```python
from build123d import *

# Parameters (mm, degrees)
SKETCH1_W           = 25
SKETCH1_H           = 30
SKETCH1_R           = 1.5
SKETCH1_R_2         = 3.5
SKETCH1_W_2         = 30
SKETCH1_H_2         = 5
BOSS_EXTRUDE4_DEPTH = 3


with BuildPart() as part:
    # Sketch1 → Boss-Extrude4 (new body)
    # profile 1 of 2: a face of its own
    with BuildSketch(Plane(origin=(0, 0, 0), x_dir=(1, 0, 0), z_dir=(0, 1, 0))):
        with Locations((-26.523048167, -1.727371577)):
            Rectangle(SKETCH1_W, SKETCH1_H)
        with Locations(Location((-18.023048167, -1.727371577, 0), (0, 0, 270))):
            Circle(SKETCH1_R, mode=Mode.SUBTRACT)
        with Locations(Location((-26.523048167, -1.727371577, 0), (0, 0, 270))):
            Circle(SKETCH1_R_2, mode=Mode.SUBTRACT)
        with Locations(Location((-35.023048167, -1.727371577, 0), (0, 0, 270))):
            Circle(SKETCH1_R, mode=Mode.SUBTRACT)
    # profile 2 of 2: a face of its own
    with BuildSketch(Plane(origin=(0, 0, 0), x_dir=(1, 0, 0), z_dir=(0, 1, 0))):
        with Locations((-26.523048167, -19.227371577)):
            Rectangle(SKETCH1_W_2, SKETCH1_H_2)
    extrude(amount=BOSS_EXTRUDE4_DEPTH)


solid = part.part
```
Could you check a few things on this model? Use its own coordinates, in mm. A direction names the side the tool comes from. Coordinates: 2 decimals unless noted, no trailing zeros. Write each loop counter-clockwise with the first axis right and the second up, starting at its lowest first coordinate (ties: lowest second). Pieces come first, ordered by that corner, then holes. Notation, with made-up numbers: (-22.75, 73.5) -> (29.25, 73.5) arc R35 cw to (29.25, 111.5) -> close; hole circle Ø2 at (80.5, 38). An arc over 180 degrees is marked (long way). Return JSON: item names as keys, results as strings.
(1) We'd pull the mould along X, two halves only. Please class faces 4 (the flat face through (-27, 1, -13.273)), 5 (the cylindrical face through (-19.487, 1.479, 1.402)), 6 (the cylindrical face through (-33.536, 1.479, 1.532)), 7 (the flat face through (-11.523, 1, 19)): +X half, -X half, draft (parallel to the pull), parting line (faces both ways), or undercut.
Numbers:
{"face 4": "draft", "face 5": "undercut", "face 6": "undercut", "face 7": "+X half"}
(2) Imagine slicing it at D-D, the plane z = -9. Please give me the cut outline in (x, y), then the cut area to 3 significant figures.
Numbers:
{"outline": "(-39.02, 0) -> (-14.02, 0) -> (-14.02, 3) -> (-39.02, 3) -> close", "area": "75.0 mm2"}
(3) I'm going to push flat-ended pins straight in: pin 1 (1.5 mm diameter, centred on y = 1, z = 7.5, fed in from +X); pin 2 (0.8 mm diameter, centred on x = -12.5, y = 1.5, fed in from -Z); pin 3 (4 mm diameter, centred on x = -26.52, z = 1.73, fed in from +Y). Where does each tip first touch, or does it pass through?
Numbers:
{"pin 1": "stops at x = -14.02", "pin 2": "stops at z = 16.73", "pin 3": "passes through"}
(4) Which directions (+Z, -Z, +X, -X, +Y, -Y) give clear straight access to the entire face, cutting with the end or side of a thin tool? Please do faces 1 (the flat face through (-40, 1, 16.727)), 2 (the flat face through (-13, 1, 16.727)), 3 (the cylindrical face through (-23.053, 1.479, 1.272)).
Numbers:
{"face 1": "-Z, -X, +Y, -Y", "face 2": "-Z, +X, +Y, -Y", "face 3": "+Y, -Y"}
(5) Imagine slicing it at C-C, the plane x = -24.5. Please give me the cut outline in (y, z), then the cut area to 3 significant figures.
Numbers:
{"outline": "(0, -13.27) -> (3, -13.27) -> (3, -1.13) -> (0, -1.13) -> close; (0, 4.58) -> (3, 4.58) -> (3, 21.73) -> (0, 21.73) -> close", "area": "87.9 mm2"}
(6) Imagine slicing it at A-A, the plane z = 4.5. Please give me the cut outline in (x, y), then the cut area to 3 significant figures.
Numbers:
{"outline": "(-39.02, 0) -> (-28.66, 0) -> (-28.66, 3) -> (-39.02, 3) -> close; (-24.39, 0) -> (-14.02, 0) -> (-14.02, 3) -> (-24.39, 3) -> close", "area": "62.2 mm2"}
(7) I need wall thicknesses on L1, parallel to Z at x = -35, y = 2.2; L2, parallel to X at y = 2.6, z = 7; L3, parallel to Z at x = -13.5, y = 1.15. Which ranges of each line are inside material? Lowest first, please.
Numbers:
{"L1": "z = -13.27 to 0.23, 3.23 to 21.73", "L2": "x = -39.02 to -14.02", "L3": "z = 16.73 to 21.73"}
(8) Imagine slicing it at B-B, the plane y = 2.4. Please give me the cut outline in (x, z), then the cut area to 3 significant figures.
Numbers:
{"outline": "(-41.52, 16.73) -> (-39.02, 16.73) -> (-39.02, -13.27) -> (-14.02, -13.27) -> (-14.02, 16.73) -> (-11.52, 16.73) -> (-11.52, 21.73) -> (-41.52, 21.73) -> close; hole circle Ø3 at (-35.02, 1.73); hole circle Ø7 at (-26.52, 1.73); hole circle Ø3 at (-18.02, 1.73)", "area": "847 mm2"}
